from build123d import *

# Parameters (mm, degrees)
EXTRUDE_2_DEPTH        = 615
SKETCH_3_R             = 3
CUT_EXTRUDE_1_DEPTH    = 3.5
SKETCH_4_R             = 1.75
CUT_EXTRUDE_2_DEPTH    = 3
PATTERN_LINEAR_1_COUNT = 30
PATTERN_LINEAR_1_PITCH = 20
FILLET_1_R             = 1


with BuildPart() as part:
    # 草图2 → 凸台-拉伸2 (new body)
    with BuildSketch(Plane.XY):
        Polygon((0, 0), (9, 0), (9, 3.5), (8.646446609, 3.853553391), (8.146446609, 3.853553391), (8.146446609, 4.353553391), (8.646446609, 4.353553391), (9, 4.707106781), (9, 6.5), (0, 6.5), (0, 4.707106781), (0.353553391, 4.353553391), (0.853553391, 4.353553391), (0.853553391, 3.853553391), (0.353553391, 3.853553391), (0, 3.5), align=None)
    extrude(amount=-EXTRUDE_2_DEPTH)

    # 草图3 → 切除-拉伸1 (cut)
    with BuildSketch(Plane(origin=(0, 6.5, 0), x_dir=(1, 0, 0), z_dir=(0, 1, 0))):
        with Locations(Location((4.5, 10, 0), (0, 0, 270))):
            Circle(SKETCH_3_R)
    cut_extrude_1 = extrude(amount=-CUT_EXTRUDE_1_DEPTH, mode=Mode.SUBTRACT)

    # 草图4 → 切除-拉伸2 (cut)
    with BuildSketch(Plane(origin=(0, 3, 0), x_dir=(1, 0, 0), z_dir=(0, 1, 0))):
        with Locations(Location((4.5, 10, 0), (0, 0, 270))):
            Circle(SKETCH_4_R)
    cut_extrude_2 = extrude(amount=-CUT_EXTRUDE_2_DEPTH, mode=Mode.SUBTRACT)

    # 阵列(线性)1: 切除-拉伸1, 切除-拉伸2 ×30
    with Locations(*[(0, 0, -i * PATTERN_LINEAR_1_PITCH) for i in range(1, PATTERN_LINEAR_1_COUNT)]):
        add(cut_extrude_1, mode=Mode.SUBTRACT)
        add(cut_extrude_2, mode=Mode.SUBTRACT)

    # 圆角1
    fillet_1_edges = [part.edges().sort_by_distance(p)[0] for p in [
        (9, 1.75, -615),
        (0, 1.75, -615),
        (9, 1.75, 0),
        (0, 1.75, 0),
    ]]
    fillet(fillet_1_edges, radius=FILLET_1_R)


solid = part.part
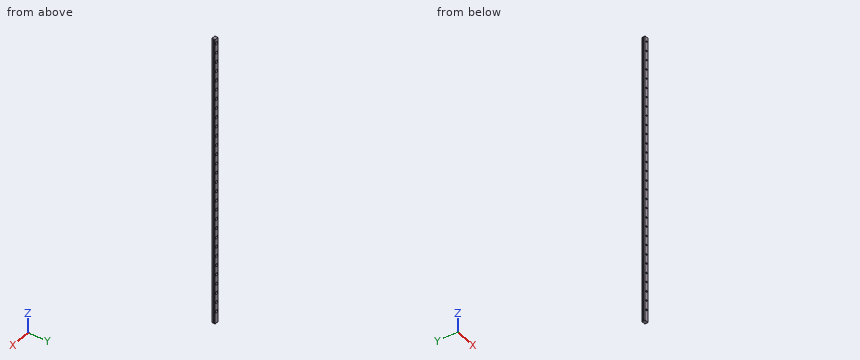
Here's how the part is built. I have some questions about the finished solid (model axes, mm). Round coordinates to 2 decimals unless told otherwise and drop trailing zeros. Order: outer loops, then holes, each group sorted by start corner. A loop starts at its lowest first (then second) coordinate and runs counter-clockwise, first axis right, second up. Notation, with made-up numbers: (69, -20.75) -> (82, -20.75) arc R28 cw to (82, -2.75) -> close; hole circle Ø9 at (20, 87.25). An arc over 180 degrees is marked (long way). Return JSON: item names as keys, results as strings.
Q1. If we section it at A-A on z = -278.5: List the corners of the cut face in (x, y) for me, plus the area to 3 significant figures.
Filled sheet:
{"outline": "(0, 0) -> (9, 0) -> (9, 3.5) -> (8.65, 3.85) -> (8.15, 3.85) -> (8.15, 4.35) -> (8.65, 4.35) -> (9, 4.71) -> (9, 6.5) -> (0, 6.5) -> (0, 4.71) -> (0.35, 4.35) -> (0.85, 4.35) -> (0.85, 3.85) -> (0.35, 3.85) -> (0, 3.5) -> close", "area": "57.4 mm^2"}
Q2. For pin 1 Ø4.5 at (x, z) = (4.5, -90) entering from +Y, with a flat end and sliding along its axis, tell me the tip position at first contact or that it passes through.
Filled sheet:
{"pin 1": "stops at y = 3"}
Q3. If we section it at B-B on y = 2: Give the number of separate pieces and of enclosed holes in the cut face, plus the area to 3 significant figures.
Filled sheet:
{"separate pieces": "1", "enclosed holes": "30", "area": "5,250 mm^2"}
Q4. I need wall thicknesses on line 1 along Y through (x, z) = (0.5, -248); line 2 along X through (y, z) = (5.1, -130); line 3 along X through (y, z) = (1.35, -510). Which ranges of each line are inside material? Lowest first, please. Write a range as from..to.
Filled sheet:
{"line 1": "y = 0..3.85, 4.35..6.5", "line 2": "x = 0..1.5, 7.5..9", "line 3": "x = 0..2.75, 6.25..9"}
